```python
from build123d import *

# Parameters (mm, degrees)
SKETCH1_W           = 90
SKETCH1_H           = 90
BOSS_EXTRUDE1_DEPTH = 2.5
SKETCH3_W           = 50
SKETCH3_H           = 50
BOSS_EXTRUDE4_DEPTH = 15
SKETCH2_W           = 40
SKETCH2_H           = 40
CUT_EXTRUDE4_DEPTH  = 2.5
SKETCH8_R           = 1.5
CUT_EXTRUDE6_DEPTH  = 5
FILLET1_R           = 2.5
FILLET2_R           = 2.5
FILLET3_R           = 2.5
SKETCH10_R          = 6.25
CUT_EXTRUDE12_DEPTH = 2.5
SKETCH11_W          = 30
SKETCH11_H          = 30
CUT_EXTRUDE13_DEPTH = 15
SKETCH12_R          = 1.5
CUT_EXTRUDE14_DEPTH = 5
FILLET4_R           = 5
FILLET5_R           = 5


with BuildPart() as part:
    # Sketch1 → Boss-Extrude1 (new body)
    with BuildSketch(Plane.XY):
        with Locations((45, 45)):
            Rectangle(SKETCH1_W, SKETCH1_H)
    extrude(amount=BOSS_EXTRUDE1_DEPTH)

    # Sketch3 → Boss-Extrude4 (add)
    with BuildSketch(Plane(origin=(0, 0, 0), x_dir=(-1, 0, 0), z_dir=(0, 0, -1))):
        with Locations((-45, 45)):
            Rectangle(SKETCH3_W, SKETCH3_H)
    extrude(amount=BOSS_EXTRUDE4_DEPTH)

    # Sketch2 → Cut-Extrude4 (cut)
    with BuildSketch(Plane.XY.offset(2.5)):
        with Locations((45, 45)):
            Rectangle(SKETCH2_W, SKETCH2_H)
    extrude(amount=-CUT_EXTRUDE4_DEPTH, mode=Mode.SUBTRACT)

    # Sketch8 → Cut-Extrude6 (cut)
    with BuildSketch(Plane.XY):
        with Locations((62, 62)):
            Circle(SKETCH8_R)
        with Locations((62, 28)):
            Circle(SKETCH8_R)
        with Locations((28, 62)):
            Circle(SKETCH8_R)
        with Locations((28, 28)):
            Circle(SKETCH8_R)
    extrude(amount=-CUT_EXTRUDE6_DEPTH, mode=Mode.SUBTRACT)

    # Fillet1
    fillet1_edges = [part.edges().sort_by_distance(p)[0] for p in [
        (0, 90, 1.25),
        (90, 90, 1.25),
        (90, 0, 1.25),
        (0, 0, 1.25),
    ]]
    fillet(fillet1_edges, radius=FILLET1_R)

    # Fillet2
    fillet2_edges = [part.edges().sort_by_distance(p)[0] for p in [
        (25, 65, 1.25),
        (65, 65, 1.25),
    ]]
    fillet(fillet2_edges, radius=FILLET2_R)

    # Fillet3
    fillet3_edges = [part.edges().sort_by_distance(p)[0] for p in [
        (25, 25, 1.25),
        (65, 25, 1.25),
    ]]
    fillet(fillet3_edges, radius=FILLET3_R)

    # Sketch10 → Cut-Extrude12 (cut)
    with BuildSketch(Plane.XY.offset(2.5)):
        with Locations((62.5, 45)):
            Circle(SKETCH10_R)
    extrude(amount=-CUT_EXTRUDE12_DEPTH, mode=Mode.SUBTRACT)

    # Sketch11 → Cut-Extrude13 (cut)
    with BuildSketch(Plane.XY):
        with Locations((45, 45)):
            Rectangle(SKETCH11_W, SKETCH11_H)
    extrude(amount=-CUT_EXTRUDE13_DEPTH, mode=Mode.SUBTRACT)

    # Sketch12 → Cut-Extrude14 (cut)
    with BuildSketch(Plane(origin=(0, 0, -15), x_dir=(-1, 0, 0), z_dir=(0, 0, -1))):
        with Locations((-28, 28)):
            Circle(SKETCH12_R)
        with Locations((-28, 62)):
            Circle(SKETCH12_R)
        with Locations((-62, 62)):
            Circle(SKETCH12_R)
        with Locations((-62, 28)):
            Circle(SKETCH12_R)
    extrude(amount=-CUT_EXTRUDE14_DEPTH, mode=Mode.SUBTRACT)

    # Fillet4
    fillet4_edges = [part.edges().sort_by_distance(p)[0] for p in [
        (70, 70, -7.5),
        (70, 20, -7.5),
    ]]
    fillet(fillet4_edges, radius=FILLET4_R)

    # Fillet5
    fillet5_edges = [part.edges().sort_by_distance(p)[0] for p in [
        (20, 20, -7.5),
        (20, 70, -7.5),
    ]]
    fillet(fillet5_edges, radius=FILLET5_R)


solid = part.part
```
Can you work these out from the model? Positions are in its coordinate system, mm. A direction names the side the tool comes from. Round coordinates to 2 decimals unless told otherwise and drop trailing zeros. Order: outer loops, then holes, each group sorted by start corner. A loop starts at its lowest first (then second) coordinate and runs counter-clockwise, first axis right, second up. Notation, with made-up numbers: (13, 28.25) -> (38, 28.25) arc R17 cw to (38, 43.25) -> close; hole circle Ø5 at (-32, -7.75). An arc over 180 degrees is marked (long way). Return JSON: item names as keys, results as strings. Group by question number.
1. If we section it at B-B, the plane x = 58: Write out the boundary of the cut face in (y, z).
2. If we section it at A-A, the plane z = -11.25: Write out the boundary of the cut face in (x, y), then the cut area to 3 significant figures.
3. Which directions (+Z, -Z, +X, -X, +Y, -Y) give clear straight access to the entire face, cutting with the end or side of a thin tool? Please do faces 5 (the face through (60.57, 62.45, -12.54)), 6 (the face through (64.287, 64.248, 1.232)), 7 (the face through (45, 60, -7)).
4. Will these pins go through, and if not, where does the flat tip stop? pin 1 (4 mm diameter, centred on y = 36, z = -6.5, fed in from -X); pin 2 (1.5 mm diameter, centred on x = 10.5, y = 77, fed in from -Z); pin 3 (7.5 mm diameter, centred on x = 38.5, z = -4.5, fed in from -Y); pin 4 (2.5 mm diameter, centred on x = 62.5, y = 28, fed in from -Z).
5. If we section it at D-D, the plane x = 23.5: Write out the boundary of the cut face in (y, z), then the cut area to 3 significant figures.
6. We'd pull the mould along Y, two halves only. Please class faces 1 (the face through (44, 76, 0)), 2 (the face through (89.248, 89.287, 1.268)), 3 (the face through (22, 21, -8)), 4 (the face through (28, 28, -10)): released by +Y, released by -Y, zero draft, split by the parting line, or undercut.
7. I need wall thicknesses on line 1 (Y direction, x = 62, z = -13.85); line 2 (X direction, y = 41.5, z = -13.25); line 3 (X direction, y = 28.5, z = -3.75). Which ranges of each line are inside material? Lowest first, please. Write a range as [from, to].
Output values:
{
 "1": {"outline": "(0, 0) -> (20, 0) -> (20, -15) -> (30, -15) -> (30, 0) -> (25, 0) -> (25, 2.5) -> (0, 2.5) -> close; (60, -15) -> (70, -15) -> (70, 0) -> (90, 0) -> (90, 2.5) -> (65, 2.5) -> (65, 0) -> (60, 0) -> close"},
 "2": {"outline": "(20, 25) arc R5 ccw to (25, 20) -> (65, 20) arc R5 ccw to (70, 25) -> (70, 65) arc R5 ccw to (65, 70) -> (25, 70) arc R5 ccw to (20, 65) -> close; hole circle Ø3 at (28, 28); hole circle Ø3 at (28, 62); hole (30, 30) -> (60, 30) -> (60, 60) -> (30, 60) -> close; hole circle Ø3 at (62, 28); hole circle Ø3 at (62, 62)", "area": "1,550 mm²"},
 "3": {"face 5": "-Z", "face 6": "+Z", "face 7": "+Z, -Z"},
 "4": {"pin 1": "x = 20", "pin 2": "z = 0", "pin 3": "y = 20", "pin 4": "z = -15"},
 "5": {"outline": "(0, 0) -> (20.23, 0) -> (20.23, -15) -> (69.77, -15) -> (69.77, 0) -> (90, 0) -> (90, 2.5) -> (0, 2.5) -> close", "area": "968 mm²"},
 "6": {"face 1": "zero draft", "face 2": "released by +Y", "face 3": "released by -Y", "face 4": "undercut"},
 "7": {"line 1": "[20, 26.5], [29.5, 60.5], [63.5, 70]", "line 2": "[20, 30], [60, 70]", "line 3": "[20, 26.59], [29.41, 60.59], [63.41, 70]"}
}
